For this review, take the finished solid that the model builds, in its own axes (mm). A direction names the side the tool comes from. Coordinates: 2 decimals unless noted, no trailing zeros. Write each loop counter-clockwise with the first axis right and the second up, starting at its lowest first coordinate (ties: lowest second). Pieces come first, ordered by that corner, then holes. Notation, with made-up numbers: (7.25, 75) -> (51.25, 75) arc R34 ccw to (51.25, 106) -> close; hole circle Ø4 at (73.25, 23). An arc over 180 degrees is marked (long way). One line per item, written item: value. Start each with the question number.
1) Add section A-A (x = 0). State the section outline as (y, z) points, and give its area (3 significant figures).
2) Machinability: for faces 4 (the flat face through (14.25, 0, 1)), 5 (the flat face through (6, 7, 1.2)), which of the approach directions +Z, -Z, +X, -X, +Y, -Y give a long, thin tool a straight path to every point of the face, cutting with its end or side? Answer none if there is none.
3) Mouldability with a two-part tool opening along X and no side actions: class faces 1 (the flat face through (-4, -5, 2.7)), 2 (the cylindrical face through (-5.894, 0.259, 1.331)), 3 (the flat face through (-14.25, 0, 1)) as released by +X, released by -X, zero draft, split by the parting line, or undercut.
4) Add section D-D (y = 10.5). State the section outline as (x, z) points, and give its area (3 significant figures).
5) For pin 1 Ø1 at (y, z) = (1.5, 2.5) entering from -X; pin 2 Ø1.5 at (y, z) = (4.5, 2) entering from -X, all flat-tipped, find the tip position at first contact; note any pin that passes through.
6) Add section C-C (z = 0.7). State the section outline as (x, y) points, and give its area (3 significant figures).
7) For probe 1 along X at (y, z) = (-0.25, 1.5); probe 2 along Y at (x, z) = (0, 1.05); probe 3 along Z at (x, y) = (-6, 5.5), list the stretches that pass through material, from the lowest coordinate up. Write a range as from..to.
from build123d import *

# Parameters (mm, degrees)
SKETCH1_W           = 28.5
SKETCH1_H           = 28.5
SKETCH1_R           = 8
SKETCH1_R_2         = 5.9
BOSS_EXTRUDE1_DEPTH = 1.2
SKETCH1_3_R         = 8
SKETCH1_3_R_2       = 5.9
BOSS_EXTRUDE2_DEPTH = 2.7
FILLET1_R           = 1


with BuildPart() as part:
    # Sketch1 → Boss-Extrude1 (new body)
    # profile 1 of 2: a face of its own
    with BuildSketch(Plane.XY):
        Rectangle(SKETCH1_W, SKETCH1_H)
        Circle(SKETCH1_R, mode=Mode.SUBTRACT)
    # profile 2 of 2: a face of its own
    with BuildSketch(Plane.XY):
        Circle(SKETCH1_R)
        Circle(SKETCH1_R_2, mode=Mode.SUBTRACT)
    extrude(amount=BOSS_EXTRUDE1_DEPTH)

    # Sketch1_3 → Boss-Extrude2 (add)
    with BuildSketch(Plane.XY):
        Circle(SKETCH1_3_R)
        Circle(SKETCH1_3_R_2, mode=Mode.SUBTRACT)
    extrude(amount=BOSS_EXTRUDE2_DEPTH)

    # Fillet1
    fillet1_edges = [part.edges().sort_by_distance(p)[0] for p in [
        (-8, 0, 2.7),
    ]]
    fillet(fillet1_edges, radius=FILLET1_R)


solid = part.part
Numbers:
1. outline: (-14.25, 0) -> (-5.9, 0) -> (-5.9, 2.7) -> (-7, 2.7) arc R1 ccw to (-8, 1.7) -> (-8, 1.2) -> (-14.25, 1.2) -> close; (5.9, 0) -> (14.25, 0) -> (14.25, 1.2) -> (8, 1.2) -> (8, 1.7) arc R1 ccw to (7, 2.7) -> (5.9, 2.7) -> close
1. area: 25.9 mm²
2. face 4: +Z, -Z, +X, +Y, -Y
2. face 5: +Z
3. face 1: zero draft
3. face 2: undercut
3. face 3: released by -X
4. outline: (-14.25, 0) -> (14.25, 0) -> (14.25, 1.2) -> (-14.25, 1.2) -> close
4. area: 34.2 mm²
5. pin 1: x = -7.83
5. pin 2: x = -7.05
6. outline: (-14.25, -14.25) -> (14.25, -14.25) -> (14.25, 14.25) -> (-14.25, 14.25) -> close; hole circle Ø11.8 at (0, 0)
6. area: 703 mm²
7. probe 1: -8..-5.89, 5.89..8
7. probe 2: -14.25..-5.9, 5.9..14.25
7. probe 3: 0..1.2
